Can you work these out from the model? Positions are in its coordinate system, mm. A direction names the side the tool comes from. Give positions to 0.01 mm unless a question says otherwise; leave off trailing zeros. Loops run counter-clockwise (first coordinate to the right, second up) from the corner with the lowest first, then second, coordinate; pieces in that order, holes last. Notation, with made-up numbers: M 61.5,52.5 L 120.5,52.5 A28 ccw 120.5,74.5 Z; hole C 16,-22.75 d8. An arc over 180 degrees is marked long. Put each result on its own line as item: value. Start each with the question number.
1) Imagine slicing it at C-C (z = -5.75). Write out the boundary of the cut face in (x, y) (3 decimals).
2) Imagine slicing it at D-D (x = -9). Write out the boundary of the cut face in (y, z).
3) For faces 1 (the cylindrical face through (4.57, 7.167, 1.775)), 2 (the flat face through (0, 12.25, -7)), which set-ups out of +Z, -Z, +X, -X, +Y, -Y let a thin tool reach every point of the face, with its end or its side?
4) For P1, Ø13.5, axis at x = -2.5, y = 1, coming from the +Z side; P2, Ø2, axis at y = -1, z = 1.5, coming from the +X side, each with a flat end and sliding along its axis, tell me the tip position at first contact or that it passes through.
5) Please list where these lines run through material, in increasing order: line 1 along Y through (x, z) = (0, -4.5) (3 decimals); line 2 along Y through (x, z) = (0, 1.2) (3 decimals); line 3 along X through (y, z) = (5.5, -7.5). Write a range as from..to.
from build123d import *

# Parameters (mm, degrees)
F0_W     = 24.5
F0_H     = 24.5
F0_R     = 8.5
F0_R_2   = 6.925
F1_DEPTH = 10
F2_DEPTH = 3.6
F3_DEPTH = 25
F4_SIZE2 = 3.74999
F4_SIZE  = 3.74999
F5_R     = 2


# Not quite as in the source:
# - a fillet or chamfer is up to 0.001 mm smaller than in the source, because OpenCascade refuses the exact size


with BuildPart() as f1:
    # F0 (on Top) → F1 (new body)
    with BuildSketch(Plane.XY):
        Rectangle(F0_W, F0_H)
        Circle(F0_R, mode=Mode.SUBTRACT)
        Circle(F0_R)
        Circle(F0_R_2, mode=Mode.SUBTRACT)
        Circle(F0_R_2)
    extrude(amount=-F1_DEPTH)

    # F0 (on Top) → F2 (join)
    with BuildSketch(Plane.XY):
        Circle(F0_R)
        Circle(F0_R_2, mode=Mode.SUBTRACT)
    extrude(amount=F2_DEPTH)

    # F0 (on Top) → F3 (cut)
    with BuildSketch(Plane.XY):
        Circle(F0_R_2)
    extrude(amount=-F3_DEPTH, mode=Mode.SUBTRACT)

    # F4 (size 3.75 and 3.75 in the source; OpenCascade refuses exactly that, so slightly less here)
    f4_edges = [f1.edges().sort_by_distance(p)[0] for p in [
        (0, -12.25, 0),
        (12.25, 0, 0),
        (0, 12.25, 0),
        (-12.25, 0, 0),
    ]]
    chamfer(f4_edges, length=F4_SIZE, length2=F4_SIZE2)

    # F5
    f5_edges = [f1.edges().sort_by_distance(p)[0] for p in [
        (12.25, -12.25, -6.874995),
        (12.25, 12.25, -6.874995),
        (-12.25, 12.25, -6.874995),
        (-12.25, -12.25, -6.874995),
    ]]
    fillet(f5_edges, radius=F5_R)


solid = f1.part
Recorded:
1. outline: M -12.25,-10.25 A2 ccw -10.25,-12.25 L 10.25,-12.25 A2 ccw 12.25,-10.25 L 12.25,10.25 A2 ccw 10.25,12.25 L -10.25,12.25 A2 ccw -12.25,10.25 Z; hole C 0,0 d13.85
2. outline: M -12.25,-10 L 12.25,-10 L 12.25,-3.75 L 9,-0.5 L -9,-0.5 L -12.25,-3.75 Z
3. face 1: +Z
3. face 2: +Z, -Z, +X, -X, +Y
4. P1: z = 3.6
4. P2: x = 8.5
5. line 1: -12.25..-6.925, 6.925..12.25
5. line 2: -8.5..-6.925, 6.925..8.5
5. line 3: -12.25..-4.21, 4.21..12.25
